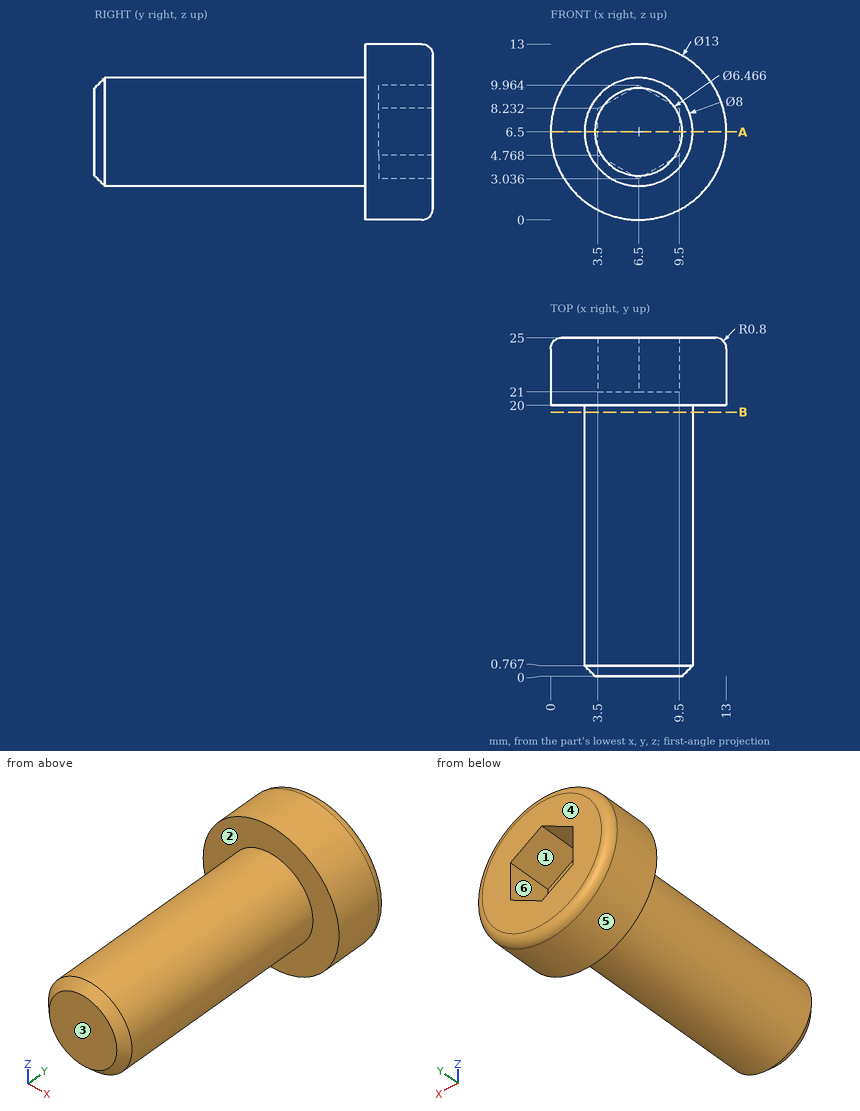
Can you work these out from the drawing? Everything is in mm from the part's minimum corner. A direction names the side the tool comes from. Round coordinates to 2 decimals unless told otherwise and drop trailing zeros. Order: outer loops, then holes, each group sorted by start corner. A loop starts at its lowest first (then second) coordinate and runs counter-clockwise, first axis right, second up.
(1) If we section it at A-A (z = 6.5): Please give me the cut outline in (x, y).
Results are:
outline: (0, 20) - (2.5, 20) - (2.5, 0.77) - (3.27, 0) - (9.73, 0) - (10.5, 0.77) - (10.5, 20) - (13, 20) - (13, 24.2) arc R0.8 ccw to (12.2, 25) - (9.5, 25) - (9.5, 21) - (3.5, 21) - (3.5, 25) - (0.8, 25) arc R0.8 ccw to (0, 24.2) - close
(2) I'm going to push flat-ended pins straight in: pin 1 (2 mm diameter, centred on x = 10, y = 11, fed in from -Z); pin 2 (1.5 mm diameter, centred on x = 2, y = 21, fed in from +Z); pin 3 (1 mm diameter, centred on x = 10.5, y = 4.5, fed in from +Z). Where does each tip first touch, or does it pass through?
Results are:
pin 1: stops at z = 3.38
pin 2: stops at z = 11.81
pin 3: stops at z = 8.44
(3) If we section it at B-B (y = 19.5): Please give me the cut outline in (x, z), plus the area to 3 significant figures.
Results are:
outline: circle Ø8 at (6.5, 6.5)
area: 50.3 mm2
(4) We'd pull the mould along Z, two halves only. Please class the marked faces 4, 5 and 6: +Z half, -Z half, draft (parallel to the pull), parting line (faces both ways), or undercut.
Results are:
face 4: draft
face 5: parting line
face 6: undercut
(5) If I drill on L1, parallel to Y at x = 2, z = 8.5; L2, parallel to X at y = 23.5, z = 6; L3, parallel to Z at x = 6.5, y = 9.5, over which ranges is the centre line in solid material (lowest first)?
Results are:
L1: y = 20 to 25
L2: x = 0.02 to 3.5, 9.5 to 12.98
L3: z = 2.5 to 10.5
(6) On a 3-axis mill with a long thin cutter (end or side, diameter ignored), from which of +Z, -Z, +X, -X, +Y, -Y can I reach the whole of each face in a straight line? I mean the marked faces 1, 2 and 3. Say none if no direction works.
Results are:
face 1: +Y
face 2: -Y
face 3: +Z, -Z, +X, -X, -Y
